Read the model definition and answer for the solid it produces. Units are mm, in the model's axes. A direction names the side the tool comes from. Coordinates: 2 decimals unless noted, no trailing zeros. Loops run counter-clockwise (first coordinate to the right, second up) from the corner with the lowest first, then second, coordinate; pieces in that order, holes last. Notation, with made-up numbers: (62, 64) -> (81, 64) arc R15 ccw to (81, 75) -> close; hole circle Ø3 at (83.5, 54.5). An arc over 180 degrees is marked (long way). Answer in a Markdown table with one row per item.
```python
from build123d import *

# Parameters (mm, degrees)
F1_DEPTH = 25.4


with BuildPart() as f1:
    # F0 (on Top) → F1 (new body)
    with BuildSketch(Plane.XY):
        with BuildLine():
            Line((0, 24.024129), (0, 37.503868))
            ThreePointArc((0, 37.503868), (-37.504638, -0.000769), (0, -37.505407))
            Line((0, -37.505407), (2.655318, -37.400453))
            Line((2.655318, -37.400453), (3.281114, -37.349965))
            Line((3.281114, -37.349965), (6.502855, -36.928073))
            Line((6.502855, -36.928073), (9.673457, -36.224913))
            Line((9.673457, -36.224913), (6.195297, -23.168214))
            Line((6.195297, -23.168214), (4.153784, -23.611279))
            Line((4.153784, -23.611279), (2.079332, -23.881992))
            Line((2.079332, -23.881992), (0, -23.970587))
            ThreePointArc((0, -23.970587), (-23.997358, 0.026771), (0, 24.024129))
        make_face()
    extrude(amount=F1_DEPTH)


solid = f1.part
```
1. A cutting plane is placed at D-D on y = -9. Give the vertices of the cut face in (x, z).
A:
| item | result |
|---|---|
| outline | (-36.41, 0) -> (-22.23, 0) -> (-22.23, 25.4) -> (-36.41, 25.4) -> close |
2. A tool of negligible diameter and unlimited length cuts with its end or side. For faces 5 (the flat face through (5.189, -23.387, 12.522)), 6 (the flat face through (4.87, -37.14, 12.52)), from which of +Z, -Z, +X, -X, +Y, -Y can it reach the whole face along a straight path? Write none if from no direction.
A:
| item | result |
|---|---|
| face 5 | +Z, -Z, +Y |
| face 6 | +Z, -Z, +X, -Y |
3. The mould has two halves that part along X. Classify faces 1 (the flat face through (-25, 1, 0)), 2 (the cylindrical face through (-37.496, 0.824, 12.522)), 3 (the flat face through (3.131, -23.745, 12.522)), 4 (the flat face through (0, 31, 13)): pulls with the +X half, pulls with the -X half, needs draft (parallel to the pull), parting line crosses it, or undercut.
A:
| item | result |
|---|---|
| face 1 | needs draft |
| face 2 | pulls with the -X half |
| face 3 | undercut |
| face 4 | pulls with the +X half |
4. Given pin 1 Ø6 at (x, z) = (-30, 19.5) entering from +Y; pin 2 Ø6.5 at (y, z) = (28, 10.5) entering from +X; pin 3 Ø10 at (y, z) = (-21.5, 13.5) entering from +X, each flat-ended and moving along its own axis, determine where each tip first touches the part or whether it passes through.
A:
| item | result |
|---|---|
| pin 1 | stops at y = 26.03 |
| pin 2 | stops at x = 0 |
| pin 3 | stops at x = 7.08 |
5. Find the intervals of material crossed by probe 1 along Y at (x, z) = (-1, 12); probe 2 along Y at (x, z) = (-19, 19.5); probe 3 along X at (y, z) = (29.5, 9.5), in increasing order.
A:
| item | result |
|---|---|
| probe 1 | y = -37.49 to -23.95, 24 to 37.49 |
| probe 2 | y = -32.34 to -14.63, 14.69 to 32.33 |
| probe 3 | x = -23.16 to 0 |
6. A cutting plane is placed at A-A on x = -18.5. Give the vertices of the cut face in (y, z), and give its area (3 significant figures).
A:
| item | result |
|---|---|
| outline | (-32.63, 0) -> (-15.26, 0) -> (-15.26, 25.4) -> (-32.63, 25.4) -> close; (15.31, 0) -> (32.62, 0) -> (32.62, 25.4) -> (15.31, 25.4) -> close |
| area | 881 mm2 |
7. A cutting plane is placed at C-C on x = -4.5. Give the vertices of the cut face in (y, z), and give its area (3 significant figures).
A:
| item | result |
|---|---|
| outline | (-37.23, 0) -> (-23.54, 0) -> (-23.54, 25.4) -> (-37.23, 25.4) -> close; (23.6, 0) -> (37.23, 0) -> (37.23, 25.4) -> (23.6, 25.4) -> close |
| area | 694 mm2 |
